Part model, mm, in its own coordinate system. Face numbers are marked on the shaded views. A direction names the side the tool comes from. Coordinates: 2 decimals unless noted, no trailing zeros. Loops run counter-clockwise (first coordinate to the right, second up) from the corner with the lowest first, then second, coordinate; pieces in that order, holes last. Notation, with made-up numbers: (28.5, 19) -> (60.5, 19) arc R18 ccw to (60.5, 31) -> close; hole circle Ø10 at (72, 13). An arc over 180 degrees is marked (long way). Use one line per item in the form item = value. Start each with the question number.
(1) Band-saw the part on B-B on x = 0. Give the cut face in (y, z).
(2) Band-saw the part on C-C on y = -0.5. Give the cut face in (x, z), then the cut area to 3 significant figures.
(3) Drill centre lines: L1, parallel to X at y = 1, z = 0; L2, parallel to Y at x = 0, z = 0; L3, parallel to Z at x = -6, y = 0. Where is each one in solid material? Low to high. Write a range as [from, to].
(4) Band-saw the part on A-A on z = 0. Give the cut face in (x, y).
(5) Pin check, flat tips, straight feed: P1, Ø2, axis at y = -1, z = -1.5, coming from the +X side; P2, Ø1.8, axis at x = -5, z = -0.5, coming from the +Y side; P3, Ø3, axis at x = 5.5, y = 1, coming from the -Z side. Stop position of each tip, or through.
(6) Band-saw the part on D-D on z = -2.25. Give the cut face in (x, y).
(7) 3-axis set-ups, long thin cutter, end or side, ignore diameter. For the marked faces 3 and 4: which of +Z, -Z, +X, -X, +Y, -Y reach the whole face in a straight line?
(8) Mould opens along X. For the marked faces 1 and 2 say: +X half, -X half, draft (parallel to the pull), parting line (faces both ways), or undercut.
```python
from build123d import *
from build123d.topology import SkipClean

# Parameters (mm, degrees)
EXTRUDE_1_DEPTH     = 3
SKETCH_2_R          = 3
EXTRUDE_2_DEPTH     = 3.25
SKETCH_3_R          = 1.75
CUT_EXTRUDE_3_DEPTH = 6.5
SKETCH_4_R          = 3.25
EXTRUDE_5_DEPTH     = 6.5
EXTRUDE_START       = 0.3
SKETCH_6_R          = 3.25
EXTRUDE_6_DEPTH     = 0.3
SKETCH_7_R          = 2.5
CUT_EXTRUDE_7_DEPTH = 16.02672619


with BuildPart() as part:
    # 草图1 → 拉伸1 (new, symmetric)
    with BuildSketch(Plane(origin=(0, 0, 0), x_dir=(1, 0, 0), z_dir=(0, 1, 0))):
        with BuildLine():
            Line((-10, -3), (10, -3))
            ThreePointArc((10, -3), (13, 0), (10, 3))
            Line((10, 3), (-10, 3))
            ThreePointArc((-10, 3), (-13, 0), (-10, -3))
        make_face()
    extrude(amount=EXTRUDE_1_DEPTH, both=True)

    # 草图2 → 拉伸2 (add, symmetric)
    with SkipClean():  # the faces are left unmerged after this step: merging them gives an invalid solid
        with BuildSketch(Plane(origin=(0, 0, 0), x_dir=(1, 0, 0), z_dir=(0, 1, 0))):
            with Locations(Location((10, 0, 0), (0, 0, 270))):
                Circle(SKETCH_2_R)
            with Locations(Location((-10, 0, 0), (0, 0, 270))):
                Circle(SKETCH_2_R)
        extrude(amount=EXTRUDE_2_DEPTH, both=True)

    # 草图3 → 拉伸3 (cut)
    with SkipClean():  # the faces are left unmerged after this step: merging them gives an invalid solid
        with BuildSketch(Plane(origin=(0, 3.25, 0), x_dir=(1, 0, 0), z_dir=(0, 1, 0))):
            with Locations(Location((-10, 0, 0), (0, 0, 270))):
                Circle(SKETCH_3_R)
            with Locations(Location((10, 0, 0), (0, 0, 270))):
                Circle(SKETCH_3_R)
        extrude(amount=-CUT_EXTRUDE_3_DEPTH, mode=Mode.SUBTRACT)

    # 草图4 → 拉伸5 (add)
    with SkipClean():  # the faces are left unmerged after this step: merging them gives an invalid solid
        with BuildSketch(Plane(origin=(0, 0, -3), x_dir=(-1, 0, 0), z_dir=(0, 0, -1))):
            Circle(SKETCH_4_R)
        extrude(amount=-EXTRUDE_5_DEPTH)

    # 草图6 → 拉伸6 (add)
    with SkipClean():  # the faces are left unmerged after this step: merging them gives an invalid solid
        with BuildSketch(Plane(origin=(0, 0, -3), x_dir=(-1, 0, 0), z_dir=(0, 0, -1)).offset(EXTRUDE_START)):
            Circle(SKETCH_6_R)
        extrude(amount=-EXTRUDE_6_DEPTH)

    # 草图7 → 拉伸7 (cut, through all)
    with SkipClean():  # the faces are left unmerged after this step: merging them gives an invalid solid
        with BuildSketch(Plane(origin=(0, 0, -3.3), x_dir=(-1, 0, 0), z_dir=(0, 0, -1))):
            Circle(SKETCH_7_R)
        extrude(amount=-CUT_EXTRUDE_7_DEPTH, mode=Mode.SUBTRACT)


solid = part.part
```
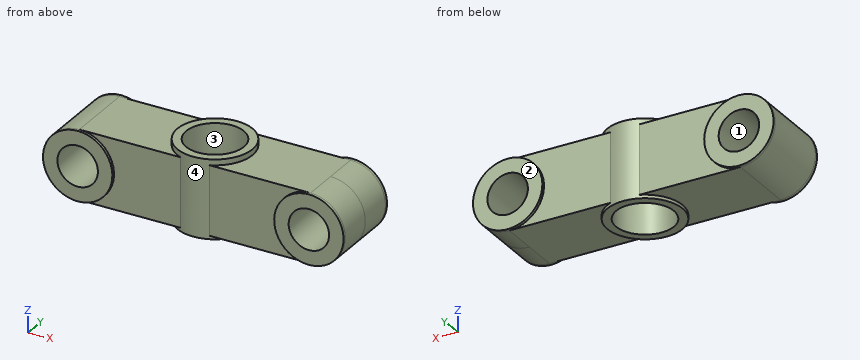
A:
q1.outline = (-3.25, -3.3) -> (-2.5, -3.3) -> (-2.5, 3.5) -> (-3.25, 3.5) -> close; (2.5, -3.3) -> (3.25, -3.3) -> (3.25, 3.5) -> (2.5, 3.5) -> close
q2.outline = (-10, -3) -> (-3.21, -3) -> (-3.21, -3.3) -> (-2.45, -3.3) -> (-2.45, 3.5) -> (-3.21, 3.5) -> (-3.21, 3) -> (-10, 3) arc R3 ccw to start; (2.45, -3.3) -> (3.21, -3.3) -> (3.21, -3) -> (10, -3) arc R3 ccw to (10, 3) -> (3.21, 3) -> (3.21, 3.5) -> (2.45, 3.5) -> close; hole circle Ø3.5 at (-10, 0); hole circle Ø3.5 at (10, 0)
q2.area = 101 mm²
q3.L1 = [-13, -11.75], [-8.25, -2.29], [2.29, 8.25], [11.75, 13]
q3.L2 = [-3.25, -2.5], [2.5, 3.25]
q3.L3 = [-3, 3]
q4.outline = (-13, -3.25) -> (-11.75, -3.25) -> (-11.75, 3.25) -> (-13, 3.25) -> close; (-8.25, -3.25) -> (-7, -3.25) -> (-7, -3) -> (-1.25, -3) arc R3.25 ccw to (1.25, -3) -> (7, -3) -> (7, -3.25) -> (8.25, -3.25) -> (8.25, 3.25) -> (7, 3.25) -> (7, 3) -> (1.25, 3) arc R3.25 ccw to (-1.25, 3) -> (-7, 3) -> (-7, 3.25) -> (-8.25, 3.25) -> close; (11.75, -3.25) -> (13, -3.25) -> (13, 3.25) -> (11.75, 3.25) -> close; hole circle Ø5 at (0, 0)
q5.P1 = 12.96
q5.P2 = 3
q5.P3 = -3
q6.outline = (-11.98, -3.25) -> (-8.02, -3.25) -> (-8.02, -3) -> (-1.25, -3) arc R3.25 ccw to (1.25, -3) -> (8.02, -3) -> (8.02, -3.25) -> (11.98, -3.25) -> (11.98, 3.25) -> (8.02, 3.25) -> (8.02, 3) -> (1.25, 3) arc R3.25 ccw to (-1.25, 3) -> (-8.02, 3) -> (-8.02, 3.25) -> (-11.98, 3.25) -> close; hole circle Ø5 at (0, 0)
q7.face_3 = +Z, -Z
q7.face_4 = none
q8.face_1 = undercut
q8.face_2 = draft
